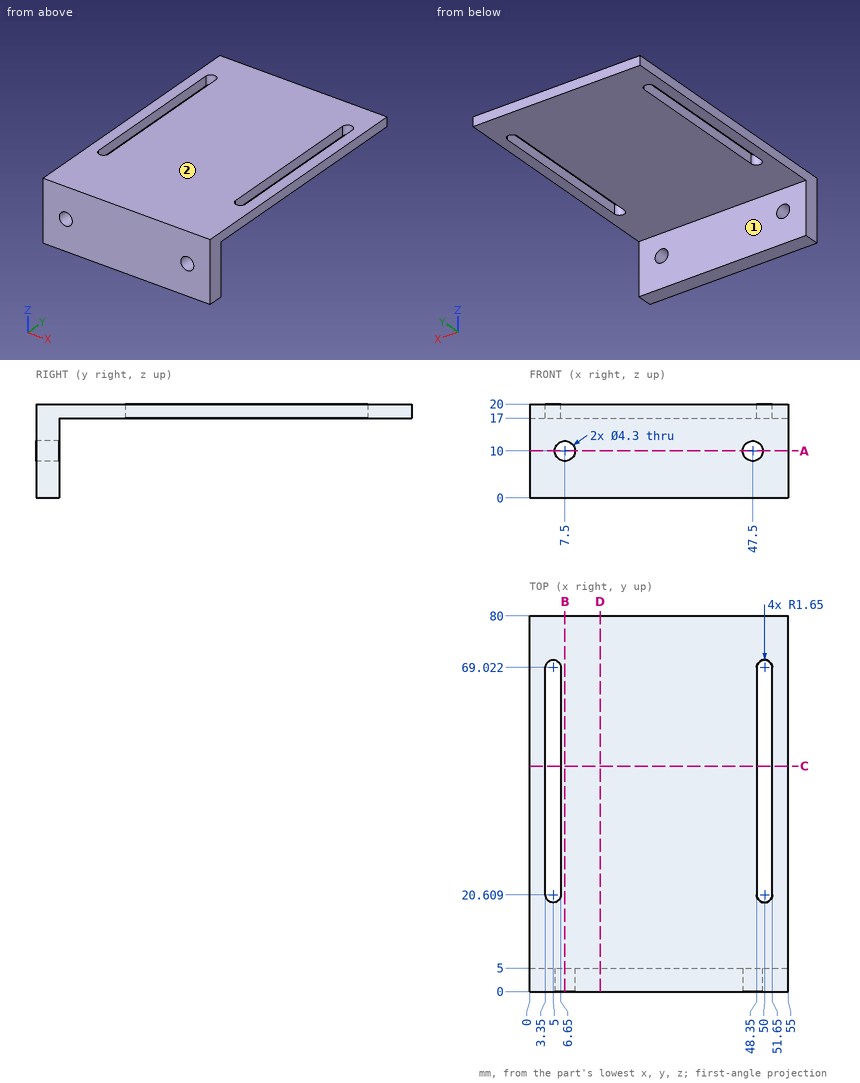
Source: three-view drawing plus pictorial views. Frame: mm from the lowest corner of the part. A direction names the side the tool comes from. Give positions to 0.01 mm unless a question says otherwise; leave off trailing zeros. Write each loop counter-clockwise with the first axis right and the second up, starting at its lowest first coordinate (ties: lowest second). Pieces come first, ordered by that corner, then holes. Notation, with made-up numbers: M 35.25,64 L 57.25,64 A25 cw 57.25,91 Z; hole C -27.5,-33 d11. An arc over 180 degrees is marked long. Use one line per item in the form item = value.
1. First-contact query: P1, Ø8.5, axis at x = 36, z = 7, coming from the +Y side; P2, Ø8, axis at x = 11.5, y = 42, coming from the -Z side. Flat tips, straight axial feed; report the tip coordinate or a pass-through.
Outcome:
P1 = 5
P2 = 17
2. Cut plane A-A on z = 10. Return loops of the section in (x, y), and give its area (3 significant figures).
Outcome:
outline = M 0,0 L 5.35,0 L 5.35,5 L 0,5 Z; M 9.65,0 L 45.35,0 L 45.35,5 L 9.65,5 Z; M 49.65,0 L 55,0 L 55,5 L 49.65,5 Z
area = 232 mm²
3. Cut plane D-D on x = 15. Return loops of the section in (y, z).
Outcome:
outline = M 0,0 L 5,0 L 5,17 L 80,17 L 80,20 L 0,20 Z
4. Ray query, L1, parallel to X at y = 3.45, z = 10; L2, parallel to Z at x = 7.5, y = 1.15; L3, parallel to Y at x = 46, z = 5.25. Return the intervals inside material, ascending.
Outcome:
L1 = 0 to 5.35, 9.65 to 45.35, 49.65 to 55
L2 = 0 to 7.85, 12.15 to 20
L3 = 0 to 5
5. Cut plane B-B on x = 7.5. Return loops of the section in (y, z).
Outcome:
outline = M 0,0 L 5,0 L 5,7.85 L 0,7.85 Z; M 0,12.15 L 5,12.15 L 5,17 L 80,17 L 80,20 L 0,20 Z
6. Cut plane C-C on y = 48. Return loops of the section in (x, z), and give its area (3 significant figures).
Outcome:
outline = M 0,17 L 3.35,17 L 3.35,20 L 0,20 Z; M 6.65,17 L 48.35,17 L 48.35,20 L 6.65,20 Z; M 51.65,17 L 55,17 L 55,20 L 51.65,20 Z
area = 145 mm²
7. Reachability of the marked faces 1 and 2 from +Z, -Z, +X, -X, +Y, -Y: full face, straight path, thin tool, end or side. Return the list, or none.
Outcome:
face_1 = -Z, +X, -X, +Y
face_2 = +Z, +X, -X, +Y, -Y
